from build123d import *

# Parameters (mm, degrees)
SKETCH_1_W          = 85
SKETCH_1_H          = 25
EXTRUDE_1_DEPTH     = 5
SKETCH_2_R          = 20
EXTRUDE_2_DEPTH     = 5
SKETCH_3_R          = 10
CUT_EXTRUDE_1_DEPTH = 35


with BuildPart() as part:
    # 草图1 → 凸台-拉伸1 (new body)
    with BuildSketch(Plane.XY):
        Rectangle(SKETCH_1_W, SKETCH_1_H)
    extrude(amount=EXTRUDE_1_DEPTH)

    # 草图2 → 凸台-拉伸2 (add)
    with BuildSketch(Plane.XY.offset(5)):
        with Locations((32.5, 0)):
            Circle(SKETCH_2_R)
        with Locations((-32.5, 0)):
            Circle(SKETCH_2_R)
    extrude(amount=-EXTRUDE_2_DEPTH)

    # 草图3 → 切除-拉伸1 (cut)
    with BuildSketch(Plane(origin=(0, 0, 0), x_dir=(-1, 0, 0), z_dir=(0, 0, -1))):
        with Locations((-32.5, 0)):
            Circle(SKETCH_3_R)
        with Locations((32.5, 0)):
            Circle(SKETCH_3_R)
    extrude(amount=-CUT_EXTRUDE_1_DEPTH, mode=Mode.SUBTRACT)


solid = part.part
Model file for the job. Use its own axes, mm. A direction names the side the tool comes from. Round coordinates to 2 decimals unless told otherwise and drop trailing zeros. Order: outer loops, then holes, each group sorted by start corner. A loop starts at its lowest first (then second) coordinate and runs counter-clockwise, first axis right, second up.
(1) Band-saw the part on B-B (x = -32.5). List the corners of the cut face in (y, z), then the cut area to 3 significant figures.
(2) Band-saw the part on A-A (y = 0). List the corners of the cut face in (x, z).
(3) 3-axis set-ups, long thin cutter, end or side, ignore diameter. For faces 1 (the face through (0, 12.5, 2)), 2 (the face through (42.49, 0.44, 2.46)), 3 (the face through (0, -12.5, 2)): which of +Z, -Z, +X, -X, +Y, -Y reach the whole face in a straight line?
(4) Band-saw the part on D-D (y = 13.5). List the corners of the cut face in (x, z).
(5) Band-saw the part on C-C (z = 2.1). List the corners of the cut face in (x, y), then the cut area to 3 significant figures.
(6) Pull direction X, two halves, no side cores. Call faces 4 (the face through (-42.04, 3, 2.46)), 5 (the face through (-1, 0, 0)), 6 (the face through (52.49, -0.69, 2.54)): released by +X, released by -X, zero draft, split by the parting line, or undercut.
(7) Pin check, flat tip, straight feed: pin 1 (1.5 mm diameter, centred on y = 1.5, z = 3, fed in from -X). Stop position of the tip, or through.
(8) Drill centre lines: line 1 (Y direction, x = 32.5, z = 1.3); line 2 (X direction, y = -1, z = 2); line 3 (X direction, y = 4.5, z = 4.1). Where is each one in solid material? Low to high.
Verdict:
1. outline: (-20, 0) - (-10, 0) - (-10, 5) - (-20, 5) - close; (10, 0) - (20, 0) - (20, 5) - (10, 5) - close
1. area: 100 mm2
2. outline: (-52.5, 0) - (-42.5, 0) - (-42.5, 5) - (-52.5, 5) - close; (-22.5, 0) - (22.5, 0) - (22.5, 5) - (-22.5, 5) - close; (42.5, 0) - (52.5, 0) - (52.5, 5) - (42.5, 5) - close
3. face 1: +Z, -Z, +Y
3. face 2: +Z, -Z
3. face 3: +Z, -Z, -Y
4. outline: (-47.26, 0) - (-17.74, 0) - (-17.74, 5) - (-47.26, 5) - close; (17.74, 0) - (47.26, 0) - (47.26, 5) - (17.74, 5) - close
5. outline: (-16.89, -12.5) - (16.89, -12.5) arc R20 ccw (long way) to (16.89, 12.5) - (-16.89, 12.5) arc R20 ccw (long way) to start; hole circle Ø20 at (-32.5, 0); hole circle Ø20 at (32.5, 0)
5. area: 2,580 mm2
6. face 4: undercut
6. face 5: zero draft
6. face 6: undercut
7. pin 1: stops at x = -52.49
8. line 1: y = -20 to -10, 10 to 20
8. line 2: x = -52.47 to -42.45, -22.55 to 22.55, 42.45 to 52.47
8. line 3: x = -51.99 to -41.43, -23.57 to 23.57, 41.43 to 51.99
